```python
from build123d import *

# Parameters (mm, degrees)
F0_R     = 4
F1_DEPTH = 6
F3_DEPTH = 25
F4_DEPTH = 120.001
F6_DEPTH = 19


with BuildPart() as f1:
    # F0 (on Top) → F1 (new body)
    with BuildSketch(Plane.XY):
        with BuildLine():
            ThreePointArc((93, 139.5), (91.681981, 142.681981), (88.5, 144))
            Line((88.5, 144), (23.5, 144))
            ThreePointArc((23.5, 144), (20.318019, 142.681981), (19, 139.5))
            ThreePointArc((19, 139.5), (17.681981, 136.318019), (14.5, 135))
            Line((14.5, 135), (4.5, 135))
            ThreePointArc((4.5, 135), (1.318019, 133.681981), (0, 130.5))
            Line((0, 130.5), (0, 4.5))
            ThreePointArc((0, 4.5), (1.318019, 1.318019), (4.5, 0))
            Line((4.5, 0), (107.5, 0))
            ThreePointArc((107.5, 0), (110.681981, 1.318019), (112, 4.5))
            Line((112, 4.5), (112, 10.5))
            ThreePointArc((112, 10.5), (110.681981, 13.681981), (107.5, 15))
            Line((107.5, 15), (19.5, 15))
            ThreePointArc((19.5, 15), (16.318019, 16.318019), (15, 19.5))
            Line((15, 19.5), (15, 115.5))
            ThreePointArc((15, 115.5), (16.318019, 118.681981), (19.5, 120))
            Line((19.5, 120), (107.5, 120))
            ThreePointArc((107.5, 120), (110.681981, 121.318019), (112, 124.5))
            Line((112, 124.5), (112, 130.5))
            ThreePointArc((112, 130.5), (110.681981, 133.681981), (107.5, 135))
            Line((107.5, 135), (97.5, 135))
            ThreePointArc((97.5, 135), (94.318019, 136.318019), (93, 139.5))
        make_face()
        with Locations((11, 129)):
            Circle(F0_R, mode=Mode.SUBTRACT)
        with Locations((36, 136)):
            Circle(F0_R, mode=Mode.SUBTRACT)
        with Locations((56, 136)):
            Circle(F0_R, mode=Mode.SUBTRACT)
        with Locations((76, 136)):
            Circle(F0_R, mode=Mode.SUBTRACT)
        with Locations((101, 129)):
            Circle(F0_R, mode=Mode.SUBTRACT)
    extrude(amount=F1_DEPTH)

    # F2 (on face) → F3 (cut)
    with BuildSketch(Plane.XZ.offset(-120)):
        with BuildLine():
            Line((21.7, 7), (21.7, 6))
            Line((21.7, 6), (24.37868, 3.32132))
            ThreePointArc((24.37868, 3.32132), (26.5, 2.442641), (28.62132, 3.32132))
            Line((28.62132, 3.32132), (31.3, 6))
            Line((31.3, 6), (41.7, 6))
            Line((41.7, 6), (44.37868, 3.32132))
            ThreePointArc((44.37868, 3.32132), (46.5, 2.442641), (48.62132, 3.32132))
            Line((48.62132, 3.32132), (51.3, 6))
            Line((51.3, 6), (61.7, 6))
            Line((61.7, 6), (64.37868, 3.32132))
            ThreePointArc((64.37868, 3.32132), (66.5, 2.442641), (68.62132, 3.32132))
            Line((68.62132, 3.32132), (71.3, 6))
            Line((71.3, 6), (81.7, 6))
            Line((81.7, 6), (84.37868, 3.32132))
            ThreePointArc((84.37868, 3.32132), (86.5, 2.442641), (88.62132, 3.32132))
            Line((88.62132, 3.32132), (91.3, 6))
            Line((91.3, 6), (91.3, 7))
            Line((91.3, 7), (21.7, 7))
        make_face()
    extrude(amount=-F3_DEPTH, mode=Mode.SUBTRACT)

    # F2 (on face) → F4 (cut, through all)
    with BuildSketch(Plane.XZ.offset(-120)):
        with BuildLine():
            Line((21.7, 7), (21.7, 6))
            Line((21.7, 6), (24.37868, 3.32132))
            ThreePointArc((24.37868, 3.32132), (26.5, 2.442641), (28.62132, 3.32132))
            Line((28.62132, 3.32132), (31.3, 6))
            Line((31.3, 6), (41.7, 6))
            Line((41.7, 6), (44.37868, 3.32132))
            ThreePointArc((44.37868, 3.32132), (46.5, 2.442641), (48.62132, 3.32132))
            Line((48.62132, 3.32132), (51.3, 6))
            Line((51.3, 6), (61.7, 6))
            Line((61.7, 6), (64.37868, 3.32132))
            ThreePointArc((64.37868, 3.32132), (66.5, 2.442641), (68.62132, 3.32132))
            Line((68.62132, 3.32132), (71.3, 6))
            Line((71.3, 6), (81.7, 6))
            Line((81.7, 6), (84.37868, 3.32132))
            ThreePointArc((84.37868, 3.32132), (86.5, 2.442641), (88.62132, 3.32132))
            Line((88.62132, 3.32132), (91.3, 6))
            Line((91.3, 6), (91.3, 7))
            Line((91.3, 7), (21.7, 7))
        make_face()
    extrude(amount=F4_DEPTH, mode=Mode.SUBTRACT)

    # F5 (on face) → F6 (join)
    with BuildSketch(Plane.XY.offset(6)):
        with BuildLine():
            Line((21.7, 5), (0, 5))
            Line((0, 5), (0, 4.5))
            ThreePointArc((0, 4.5), (1.318019, 1.318019), (4.5, 0))
            Line((4.5, 0), (21.7, 0))
            Line((21.7, 0), (21.7, 5))
        make_face()
        with BuildLine():
            Line((91.3, 5), (91.3, 0))
            Line((91.3, 0), (107.5, 0))
            ThreePointArc((107.5, 0), (110.681981, 1.318019), (112, 4.5))
            Line((112, 4.5), (112, 10.5))
            ThreePointArc((112, 10.5), (110.681981, 13.681981), (107.5, 15))
            Line((107.5, 15), (99, 15))
            Line((99, 15), (99, 5))
            Line((99, 5), (91.3, 5))
        make_face()
        with BuildLine():
            Line((107.5, 135), (99, 135))
            Line((99, 135), (99, 120))
            Line((99, 120), (107.5, 120))
            ThreePointArc((107.5, 120), (110.681981, 121.318019), (112, 124.5))
            Line((112, 124.5), (112, 130.5))
            ThreePointArc((112, 130.5), (110.681981, 133.681981), (107.5, 135))
        make_face()
    extrude(amount=F6_DEPTH)


solid = f1.part
```
The model under review builds one solid part; all positions refer to its coordinate system, in mm. A direction names the side the tool comes from. Round coordinates to 2 decimals unless told otherwise and drop trailing zeros. Order: outer loops, then holes, each group sorted by start corner. A loop starts at its lowest first (then second) coordinate and runs counter-clockwise, first axis right, second up. Notation, with made-up numbers: (-22.5, -23) -> (29.5, -23) arc R21 cw to (29.5, 15) -> close; hole circle Ø11 at (3.5, 81.5). An arc over 180 degrees is marked (long way). One line per item, written item: value. Start each with the question number.
Q1. Take a section at A-A (y = 129). Count the separate pieces of the cut face and the enclosed holes in it, and give its area (3 significant figures).
Q2. Clearance check with flat-ended pins moving along their axes: pin 1 Ø1.8 at (x, y) = (102, 130.5) entering from -Z; pin 2 Ø6 at (x, y) = (93.5, 8.5) entering from +Z; pin 3 Ø11 at (y, z) = (9, 13) entering from -X; pin 4 Ø2.5 at (x, z) = (94, 15.5) entering from +Y. State where each tip first meets the part, or that it passes through.
Q3. Take a section at B-B (x = 36). Write out the cut boundary in (y, z), and give its area (3 significant figures).
Q4. Machinability: for faces 1 (the face through (78, 132, 6)), 2 (the face through (103.15, 132.373, 2.958)), 3 (the face through (94, 129, 6)), 4 (the face through (77, 15, 4)), 5 (the face through (91.3, 3, 15)), which of the approach directions +Z, -Z, +X, -X, +Y, -Y give a long, thin tool a straight path to every point of the face, cutting with its end or side? Answer none if there is none.
Q5. Take a section at D-D (x = 11). Write out the cut boundary in (y, z).
Q6. Wall thickness on line 1 (Y direction, x = 101, z = 1.75); line 2 (Y direction, x = 36.5, z = 3.5); line 3 (Y direction, x = 100, z = 17): over which ranges is each line inside the solid? List them lowest first.
Q7. Take a section at C-C (z = 16). Write out the cut boundary in (x, y), and give its area (3 significant figures).
Q8. Mouldability with a two-part tool opening along X and no side actions: class faces 6 (the face through (56, 8, 6)), 7 (the face through (1.283, 1.353, 12.325)), 8 (the face through (103, 135, 12)) as released by +X, released by -X, zero draft, split by the parting line, or undercut.
Reported:
1. separate pieces: 3
1. enclosed holes: 0
1. area: 739 mm2
2. pin 1: stops at z = 6
2. pin 2: stops at z = 6
2. pin 3: stops at x = 0
2. pin 4: stops at y = 5
3. outline: (0, 0) -> (15, 0) -> (15, 6) -> (0, 6) -> close; (120, 0) -> (132, 0) -> (132, 6) -> (120, 6) -> close; (140, 0) -> (144, 0) -> (144, 6) -> (140, 6) -> close
3. area: 186 mm2
4. face 1: +Z, -X, +Y, -Y
4. face 2: -Z
4. face 3: +Z, -X, +Y
4. face 4: +Z, -Z, +X
4. face 5: +Z, +Y, -Y
5. outline: (0, 0) -> (125, 0) -> (125, 6) -> (5, 6) -> (5, 25) -> (0, 25) -> close; (133, 0) -> (135, 0) -> (135, 6) -> (133, 6) -> close
6. line 1: y = 0 to 15, 120 to 125, 133 to 135
6. line 2: y = 0 to 15, 120 to 132.03, 139.97 to 144
6. line 3: y = 0 to 15, 120 to 135
7. outline: (0, 4.5) arc R4.5 ccw to (4.5, 0) -> (21.7, 0) -> (21.7, 5) -> (0, 5) -> close; (91.3, 0) -> (107.5, 0) arc R4.5 ccw to (112, 4.5) -> (112, 10.5) arc R4.5 ccw to (107.5, 15) -> (99, 15) -> (99, 5) -> (91.3, 5) -> close; (99, 120) -> (107.5, 120) arc R4.5 ccw to (112, 124.5) -> (112, 130.5) arc R4.5 ccw to (107.5, 135) -> (99, 135) -> close
7. area: 515 mm2
8. face 6: undercut
8. face 7: released by -X
8. face 8: zero draft
